Autodesk Inventor part; units mm, degrees
ref_plane "YZ Plane" through (0, 0, 0) normal (1, 0, 0) x (0, 1, 0)
ref_plane "XZ Plane" through (0, 0, 0) normal (0, 1, 0) x (-1, 0, 0)
ref_plane "XY Plane" through (0, 0, 0) normal (0, 0, 1) x (1, 0, 0)
sketch "Sketch3" plane through (0, 0, 0) normal (0, 1, 0) x (-1, 0, 0)
  circle A0 centre (0, 0) radius 4.5
  circle A1 centre (0, 0) radius 2.6
  dimension "d10" = 9
  dimension "d11" = 5.2
extrude "Extrusion2" add sketch "Sketch3" along normal blind 4
sketch "Sketch4" plane through (0, 4, 0) normal (0, 1, 0) x (1, 0, 0)
  circle A0 centre (0, 0) radius 2.6
  line L0 (0, -2.6) -> (0, -1.6)
  line L1 (0, -1.6) -> (0, 2.6)
  line L2 (0, -1.6) -> (-2.0494, -1.6)
  line L3 (0, -1.6) -> (2.0494, -1.6)
  line L4 (0, 2.6) -> (0, 2.6)
  line L5 (0, 2.6) -> (0, 2.6)
  circle A1 centre (0, 0) radius 4.5
  circle A2 centre (0, 0) radius 2.6
  line L6 (0, 2.6) -> (0, 1.6)
  line L7 (0, 1.6) -> (2.0494, 1.6)
  line L8 (0, 1.6) -> (-2.0494, 1.6)
  point P0 (2.0494, 1.6)
  point P1 (-2.0494, 1.6)
  dimension "d14" = 1
  dimension "d20" = 1
extrude "Extrusion3" add sketch "Sketch4" along normal blind 6 contours L7 L1 A0 | A0 L0 L3 | L1 L8 A0 | A0 L2 L0 | A1
sketch "Sketch5" plane through (0, 10, 0) normal (0, 1, 0) x (1, 0, 0)
  circle A0 centre (0, 0) radius 4.5
extrude "Extrusion4" add sketch "Sketch5" along normal blind 1
sketch "Sketch6" plane through (2.0494, 4, 1.6) normal (0, 0, -1) x (-1, 0, 0)
  line L0 (4.0988, 6) -> (0, 6)
  line L1 (2.0494, 6) -> (2.0494, 3)
  line L2 (2.0494, 6) -> (5.0494, 6) construction
  line L3 (2.0494, 6) -> (-0.9506, 6)
  line L4 (2.0494, 6) -> (5.0494, 6) construction
  line L5 (-0.9506, 6) -> (-0.9506, 0)
  line L6 (-0.9506, 0) -> (5.0494, 0)
  line L7 (5.0494, 0) -> (5.0494, 6)
  line L8 (5.0494, 6) -> (-0.9506, 6)
  line L9 (4.6494, 6) -> (4.6494, -4)
  point P0 (2.0494, -4)
  point P1 (4.6494, 0)
  point P2 (0, 6)
  dimension "d21" = 3
  dimension "d22" = 90
  dimension "d32" = 3
  dimension "d33" = 180
  dimension "d34" = 6
  dimension "d35" = 90
  dimension "d36" = 6
  dimension "d37" = 90
extrude "Extrusion7" add sketch "Sketch6" against normal blind 46.2 contours L8 L9 L6 L5 L3 L0
sketch "Sketch8" plane through (3, 4, 3.3541) normal (1, 0, 0) x (0, 0, -1)
  line L0 (-0.3188, 6) -> (-44.4459, 6)
  line L1 (-44.4459, 6) -> (-38.4459, 6)
  line L2 (-38.4459, 6) -> (-38.4459, 0)
  line L3 (-0.3188, 0) -> (-44.4459, 0)
  line L4 (0, 6) -> (0, 0)
  line L5 (0, 6) -> (-44.4459, 6)
  line L6 (-44.4459, 0) -> (-44.4459, 6)
  line L7 (0, 0) -> (-44.4459, 0)
  point P0 (3.3541, -4)
  dimension "d40" = 6
extrude "Extrusion8" add sketch "Sketch8" along normal blind 35.56 contours L2 L3 L6 L0
sketch "Sketch11" plane through (38.56, 4, 3.3541) normal (1, 0, 0) x (0, 0, -1)
  line L0 (-44.4459, 6) -> (-44.4459, 0)
  line L1 (-44.4459, 6) -> (-51.4436, 6)
  line L2 (-51.4436, 6) -> (-51.4436, 13.0104)
  line L3 (-51.4436, 13.0104) -> (-44.4459, 13.0104)
  line L4 (-44.4459, 13.0104) -> (-44.4459, 6)
  line L5 (-51.4436, 13.0104) -> (-31.4538, 13.0104)
  line L6 (-31.4538, 13.0104) -> (-31.4538, -6.9794)
  line L7 (-31.4538, -6.9794) -> (-51.4436, -6.9794)
  line L8 (-51.4436, -6.9794) -> (-51.4436, 13.0104)
  point P0 (3.3541, -4)
  dimension "d59" = 6.9977
  dimension "d60" = 7.0104
  dimension "d61" = 19.9898
  dimension "d62" = 19.9898
extrude "Extrusion11" add sketch "Sketch11" along normal blind 3
properties part number "socket"
Geometry check sheet. Reference: the model listing, model coordinates, mm. A direction names the side the tool comes from. Give positions to 0.01 mm unless a question says otherwise; leave off trailing zeros. Order: outer loops, then holes, each group sorted by start corner. A loop starts at its lowest first (then second) coordinate and runs counter-clockwise, first axis right, second up.
1. Sectioned sample at C-C (y = 6.75). Record the boundary of the cut face in (x, z), then the cut area to 3 significant figures.
Completed:
outline: (-2.6, 3.67) arc R4.5 ccw (long way) to (3, 3.35) - (3, 41.8) - (38.56, 41.8) - (38.56, 34.81) - (41.56, 34.81) - (41.56, 54.8) - (38.56, 54.8) - (38.56, 47.8) - (-2.6, 47.8) - close; hole (-2.05, -1.6) - (2.05, -1.6) arc R2.6 ccw to (2.05, 1.6) - (-2.05, 1.6) arc R2.6 ccw to start
area: 566 mm2
2. Draft check along Z on faces 1 (the face through (0, 10, 0)), 2 (the face through (-2.6, 7, 25)), 3 (the face through (40, 7, 34.808)). Enter one of: pulls with the +Z half, pulls with the -Z half, needs draft (parallel to the pull), parting line crosses it, or undercut.
Completed:
face 1: undercut
face 2: needs draft
face 3: pulls with the -Z half
3. Scan lines: line 1 (Z direction, x = 0, y = 8); line 2 (X direction, y = 5.75, z = 0); line 3 (Z direction, x = 4, y = 8.5). Record each from-to range of solid material in increasing order.
Completed:
line 1: z = -4.5 to -1.6, 1.6 to 47.8
line 2: x = -4.5 to -2.6, 2.6 to 4.5
line 3: z = -2.06 to 2.06, 41.8 to 47.8
4. Sectioned sample at A-A (z = 38). Record the boundary of the cut face in (x, y).
Completed:
outline: (-2.6, 4) - (3, 4) - (3, 10) - (-2.6, 10) - close; (38.56, -2.98) - (41.56, -2.98) - (41.56, 17.01) - (38.56, 17.01) - close
5. Sectioned sample at D-D (z = 17). Record the boundary of the cut face in (x, y).
Completed:
outline: (-2.6, 4) - (3, 4) - (3, 10) - (-2.6, 10) - close
6. Access from +Z, -Z, +X, -X, +Y, -Y to the whole of each face (thin tool, end or side, straight path). Record for faces 4 (the face through (0, 7, -1.6)), 5 (the face through (18, 7, 47.8)), 6 (the face through (38.56, 7, 49)), 7 (the face through (40, 17.01, 45)), 8 (the face through (3, 7, 22)).
Completed:
face 4: -Y
face 5: +Z, -X, +Y, -Y
face 6: none
face 7: +Z, -Z, +X, -X, +Y
face 8: +Y, -Y
7. Depth check by flat-ended pin: pin 1 (0.5 mm diameter, centred on x = 0.5, z = 2, fed in from -Y); pin 2 (2 mm diameter, centred on x = -1, y = 8, fed in from +Z); pin 3 (3 mm diameter, centred on y = 7.5, z = 18, fed in from -X); pin 4 (1.5 mm diameter, centred on x = 7.5, y = 1.5, fed in from +Z). Enter the tip coordinate at first touch or a pass-through.
Completed:
pin 1: stops at y = 4
pin 2: stops at z = 47.8
pin 3: stops at x = -2.6
pin 4: passes through
8. Sectioned sample at B-B (y = 3.25). Record the boundary of the cut face in (x, z).
Completed:
outline: circle Ø9 at (0, 0); (38.56, 34.81) - (41.56, 34.81) - (41.56, 54.8) - (38.56, 54.8) - close; hole circle Ø5.2 at (0, 0)
